Model file for the job. Use its own axes, mm. Face numbers are marked on the shaded views. A direction names the side the tool comes from. Round coordinates to 2 decimals unless told otherwise and drop trailing zeros. Order: outer loops, then holes, each group sorted by start corner. A loop starts at its lowest first (then second) coordinate and runs counter-clockwise, first axis right, second up. Notation, with made-up numbers: M 11,57.5 L 26,57.5 A22 cw 26,84.5 Z; hole C 23,-36 d5. An arc over 180 degrees is marked long. Return JSON: item names as keys, results as strings. Group by question number.
Item 1: Slice it at B-B on y = 30.5. Write the cut outline in (x, z).
Item 2: Probe line 1 along Y through (x, z) = (-1.5, -1.5); line 2 along X through (y, z) = (29, -5.25); line 3 along Z through (x, y) = (-1.5, 31). List the from-to ranges inside material, lowest first.
Item 3: Pull direction Z, two halves, no side cores. Call the marked faces 3, 4, 5 and 6: pulls with the +Z half, pulls with the -Z half, needs draft (parallel to the pull), parting line crosses it, or undercut.
Item 4: Pin check, flat tips, straight feed: pin 1 Ø1.5 at (x, y) = (3.5, 20.5) entering from +Z; pin 2 Ø3 at (x, y) = (-4, 8) entering from +Z; pin 3 Ø6 at (y, z) = (24.5, -5) entering from -X. Stop position of each tip, or through.
Item 5: Which spindle directions (+Z, -Z, +X, -X, +Y, -Y) get a long thin tool onto all of the face, cutting with end or side? Do the marked faces 1 and 2. Say none if no direction does.
Item 6: Slice it at A-A on y = 27. Write the cut outline in (x, z), then the cut area to 3 significant figures.
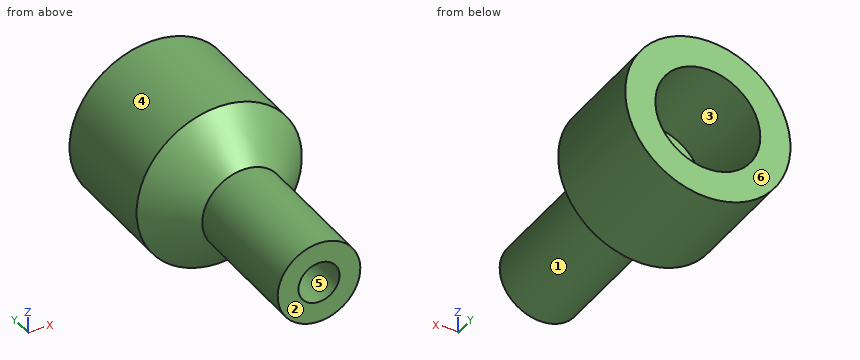
from build123d import *

# Parameters (mm, degrees)
SKETCH1_R           = 5.08
BOSS_EXTRUDE1_DEPTH = 20.8
SKETCH2_R           = 10.16
BOSS_EXTRUDE2_DEPTH = 13.97
SKETCH4_R           = 6.052157879
SKETCH3_R           = 6.450000054
CHAMFER1_SIZE       = 5.08
SKETCH6_R           = 2.325
SKETCH5_R           = 2.525


with BuildPart() as part:
    # Sketch1 → Boss-Extrude1 (new body)
    with BuildSketch(Plane(origin=(0, 0, 0), x_dir=(1, 0, 0), z_dir=(0, 1, 0))):
        with Locations(Location((0, 0, 0), (0, 0, 270))):
            Circle(SKETCH1_R)
    extrude(amount=BOSS_EXTRUDE1_DEPTH)

    # Sketch2 → Boss-Extrude2 (add)
    with BuildSketch(Plane(origin=(0, 20.8, 0), x_dir=(1, 0, 0), z_dir=(0, 1, 0))):
        with Locations(Location((0, 0, 0), (0, 0, 270))):
            Circle(SKETCH2_R)
    extrude(amount=BOSS_EXTRUDE2_DEPTH)

    # Sketch4 → Cut-Loft1 section 0
    with BuildSketch(Plane(origin=(0, 23.34, 0), x_dir=(-1, 0, 0), z_dir=(0, -1, 0))):
        Circle(SKETCH4_R)
    # Sketch3 → Cut-Loft1 section 1
    with BuildSketch(Plane(origin=(0, 34.77, 0), x_dir=(1, 0, 0), z_dir=(0, 1, 0))):
        Circle(SKETCH3_R)
    loft(mode=Mode.SUBTRACT)

    # Chamfer1
    chamfer1_edges = [part.edges().sort_by_distance(p)[0] for p in [
        (0, 20.8, -5.08),
    ]]
    chamfer(chamfer1_edges, length=CHAMFER1_SIZE - 0.0001)  # a hair under: the kernel refuses the full size

    # Sketch6 → Cut-Loft2 section 0
    with BuildSketch(Plane(origin=(0, 18.26, 0), x_dir=(-1, 0, 0), z_dir=(0, -1, 0))):
        Circle(SKETCH6_R)
    # Sketch5 → Cut-Loft2 section 1
    with BuildSketch(Plane.XZ):
        Circle(SKETCH5_R)
    loft(mode=Mode.SUBTRACT)


solid = part.part
Output values:
{
 "1": {"outline": "C 0,0 d20.32; hole C 0,0 d12.6"},
 "2": {"line 1": "18.26 to 23.34", "line 2": "-8.7 to -3.39, 3.39 to 8.7", "line 3": "-10.05 to -6.14, 6.14 to 10.05"},
 "3": {"face 3": "undercut", "face 4": "parting line crosses it", "face 5": "undercut", "face 6": "needs draft"},
 "4": {"pin 1": "z = 9.76", "pin 2": "z = 4.42", "pin 3": "x = -9.96"},
 "5": {"face 1": "-Y", "face 2": "+Z, -Z, +X, -X, -Y"},
 "6": {"outline": "C 0,0 d20.32; hole C 0,0 d12.36", "area": "204 mm²"}
}
